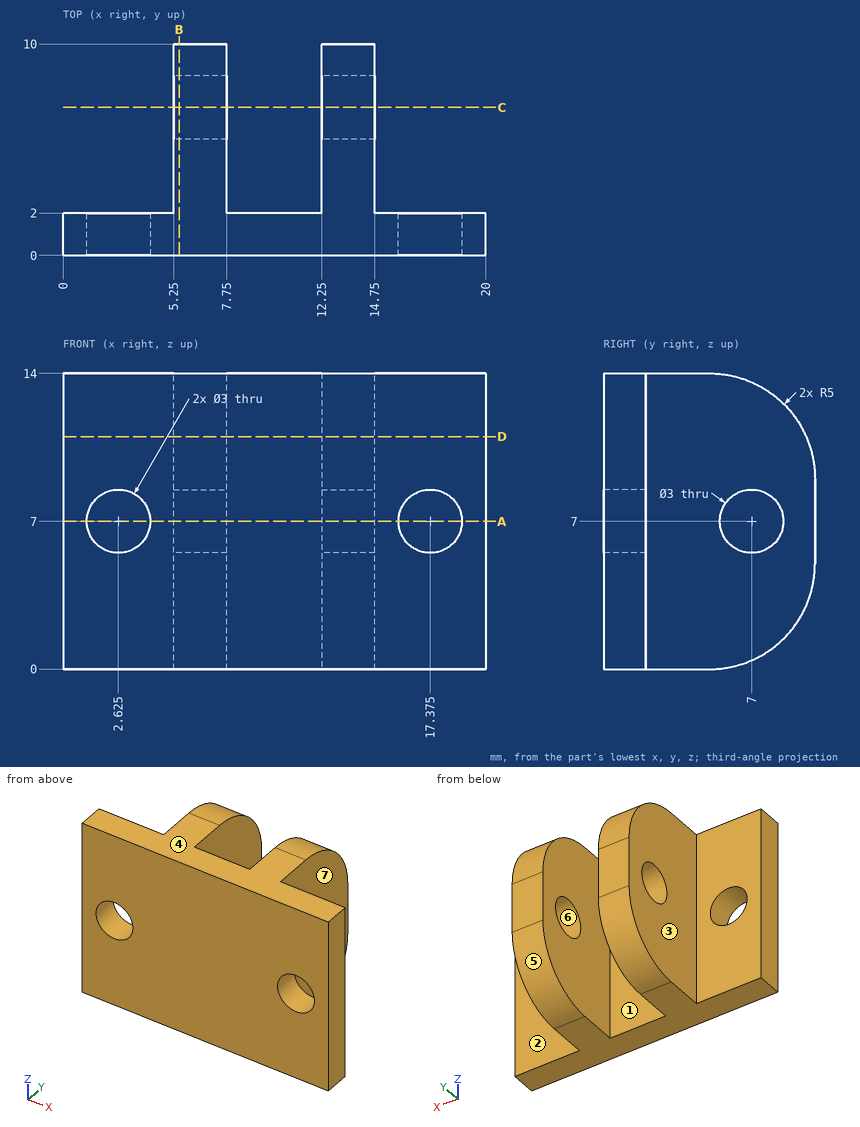
Geometry: see drawing. Coordinates: mm, zero at the bounding-box minimum. A direction names the side the tool comes from. Round coordinates to 2 decimals unless told otherwise and drop trailing zeros. Write each loop counter-clockwise with the first axis right and the second up, starting at its lowest first coordinate (ties: lowest second). Pieces come first, ordered by that corner, then holes. Notation, with made-up numbers: (-14.75, 54) - (39.25, 54) arc R18 ccw to (39.25, 74) - close; hole circle Ø6 at (-26.75, 16.25). An arc over 180 degrees is marked (long way). Use CSV: the item, a comma, the result in double quotes. Start each with the question number.
(1) Cut plane A-A, the plane z = 7. Return loops of the section in (x, y) (3 decimals).
(2) Cut plane B-B, the plane x = 5.5. Return loops of the section in (y, z).
(3) Material intervals for probe 1 along X at (y, z) = (9.75, 6.5); probe 2 along Y at (x, z) = (7.25, 7); probe 3 along Z at (x, y) = (18.25, 1.5), sorted ascending. Write a range as [from, to].
(4) Cut plane C-C, the plane y = 7. Return loops of the section in (x, z).
(5) Set-up query: the marked faces 1, 2 and 3. Return all of +Z, -Z, +X, -X, +Y, -Y with unobstructed straight access to the full face (end or side cutting, diameter ignored); none if empty.
(6) Cut plane D-D, the plane z = 11. Return loops of the section in (x, y), and give its area (3 significant figures).
(7) First-contact query: pin 1 Ø4 at (y, z) = (5.5, 5) entering from +X; pin 2 Ø3.5 at (x, z) = (2.625, 7) entering from +Y; pin 3 Ø3.5 at (y, z) = (7, 7) entering from -X. Flat tips, straight axial feed; report the tip coordinate or a pass-through.
(8) Mould query, pull axis Z, two halves, no side actions, for the marked faces 4, 5, 6 and 7. Classes: pulls with the +Z half, pulls with the -Z half, needs draft (parallel to the pull), parting line crosses it, or undercut.
Geometry says:
1,outline,"(0, 0) - (1.125, 0) - (1.125, 2) - (0, 2) - close; (4.125, 0) - (15.875, 0) - (15.875, 2) - (14.75, 2) - (14.75, 5.5) - (12.25, 5.5) - (12.25, 2) - (7.75, 2) - (7.75, 5.5) - (5.25, 5.5) - (5.25, 2) - (4.125, 2) - close; (5.25, 8.5) - (7.75, 8.5) - (7.75, 10) - (5.25, 10) - close; (12.25, 8.5) - (14.75, 8.5) - (14.75, 10) - (12.25, 10) - close; (18.875, 0) - (20, 0) - (20, 2) - (18.875, 2) - close"
2,outline,"(0, 0) - (5, 0) arc R5 ccw to (10, 5) - (10, 9) arc R5 ccw to (5, 14) - (0, 14) - close; hole circle Ø3 at (7, 7)"
3,probe 1,"[5.25, 7.75], [12.25, 14.75]"
3,probe 2,"[0, 5.5], [8.5, 10]"
3,probe 3,"[0, 5.78], [8.22, 14]"
4,outline,"(5.25, 0.42) - (7.75, 0.42) - (7.75, 5.5) - (5.25, 5.5) - close; (5.25, 8.5) - (7.75, 8.5) - (7.75, 13.58) - (5.25, 13.58) - close; (12.25, 0.42) - (14.75, 0.42) - (14.75, 5.5) - (12.25, 5.5) - close; (12.25, 8.5) - (14.75, 8.5) - (14.75, 13.58) - (12.25, 13.58) - close"
5,face 1,"+Z, -Z, +Y"
5,face 2,"+Z, -Z, +X, +Y"
5,face 3,"+Z, -Z, -X, +Y"
6,outline,"(0, 0) - (20, 0) - (20, 2) - (14.75, 2) - (14.75, 9.58) - (12.25, 9.58) - (12.25, 2) - (7.75, 2) - (7.75, 9.58) - (5.25, 9.58) - (5.25, 2) - (0, 2) - close"
6,area,"77.9 mm²"
7,pin 1,"x = 14.75"
7,pin 2,"y = 2"
7,pin 3,"x = 5.25"
8,face 4,"pulls with the +Z half"
8,face 5,"pulls with the -Z half"
8,face 6,"undercut"
8,face 7,"needs draft"
